```python
from build123d import *

# Parameters (mm, degrees)
SKETCH_W        = 23.25
SKETCH_H        = 34.68
PAD_DEPTH       = 10.5
SKETCH001_R     = 1.5
PAD001_DEPTH    = 2
SKETCH002_R     = 1.75
SKETCH002_R_2   = 2
SKETCH002_R_3   = 1
POCKET_DEPTH    = 1
FILLET_R        = 2.5
FILLET001_R     = 0.75
SKETCH003_W     = 5.08
SKETCH003_H     = 2.54
POCKET001_DEPTH = 5
SKETCH004_W     = 0.6
SKETCH004_H     = 0.6
SKETCH004_W_2   = 6.69
PAD002_DEPTH    = 4
SKETCH005_W     = 19.75
SKETCH005_H     = 31.18
POCKET002_DEPTH = 0.5
SKETCH006_W     = 4
SKETCH006_H     = 2.75
PAD003_DEPTH    = 2


with BuildPart() as part:
    # Sketch → Pad (new body)
    with BuildSketch(Plane.XY):
        Rectangle(SKETCH_W, SKETCH_H)
    extrude(amount=PAD_DEPTH)

    # Sketch001 (on Face5 of Pad) → Pad001 (join)
    with BuildSketch(Plane(origin=(0, 0, 0), x_dir=(1, 0, 0), z_dir=(0, 0, -1))):
        with BuildLine():
            Line((-11.625, 20.34), (-11.625, 17.34))
            Line((-11.625, 17.34), (-5.625, 17.34))
            Line((-5.625, 17.34), (-5.625, 20.34))
            ThreePointArc((-5.625, 20.34), (-8.625, 23.34), (-11.625, 20.34))
        make_face()
        with Locations((-8.625, 20.34)):
            Circle(SKETCH001_R, mode=Mode.SUBTRACT)
        with BuildLine():
            Line((5.625, 20.34), (5.625, 17.34))
            Line((5.625, 17.34), (11.625, 17.34))
            Line((11.625, 17.34), (11.625, 20.34))
            ThreePointArc((11.625, 20.34), (8.625, 23.34), (5.625, 20.34))
        make_face()
        with Locations((8.625, 20.34)):
            Circle(SKETCH001_R, mode=Mode.SUBTRACT)
    extrude(amount=-PAD001_DEPTH)

    # Sketch002 (on Face2 of Pad001) → Pocket (cut)
    with BuildSketch(Plane.XY.offset(10.5)):
        with Locations((0, 12.24)):
            Circle(SKETCH002_R)
        with Locations((0, 2.24)):
            Circle(SKETCH002_R_2)
        with Locations((0, 2.24)):
            Circle(SKETCH002_R_3, mode=Mode.SUBTRACT)
    extrude(amount=-POCKET_DEPTH, mode=Mode.SUBTRACT)

    # Fillet
    fillet_edges = [part.edges().sort_by_distance(p)[0] for p in [
        (11.625, -17.34, 6.25),
        (-11.625, -17.34, 6.25),
        (11.625, 17.34, 5.25),
        (-11.625, 17.34, 5.25),
    ]]
    fillet(fillet_edges, radius=FILLET_R)

    # Fillet001
    fillet001_edges = [part.edges().sort_by_distance(p)[0] for p in [
        (11.625, 0, 10.5),
        (10.892767, -16.607767, 10.5),
        (0, -17.34, 10.5),
        (-10.892767, -16.607767, 10.5),
        (-11.625, 0, 10.5),
        (-10.892767, 16.607767, 10.5),
        (0, 17.34, 10.5),
        (10.892767, 16.607767, 10.5),
        (-10.892767, 16.607767, 0),
        (-11.625, -18.84, 2),
        (-8.625, -23.34, 2),
        (-5.625, -18.84, 2),
        (5.625, -18.84, 2),
        (8.625, -23.34, 2),
        (11.625, -18.84, 2),
    ]]
    fillet(fillet001_edges, radius=FILLET001_R)

    # Sketch003 (on Face41 of Fillet001) → Pocket001 (cut)
    with BuildSketch(Plane(origin=(0, 17.34, 0), x_dir=(-1, 0, 0), z_dir=(0, 1, 0))):
        with Locations((-5.585, 5.25)):
            Rectangle(SKETCH003_W, SKETCH003_H)
        with BuildLine():
            ThreePointArc((1.61, 6.575), (0.285, 5.25), (1.61, 3.925))
            Line((1.61, 3.925), (7.3, 3.925))
            ThreePointArc((7.3, 3.925), (8.625, 5.25), (7.3, 6.575))
            Line((1.61, 6.575), (7.3, 6.575))
        make_face()
    extrude(amount=-POCKET001_DEPTH, mode=Mode.SUBTRACT)

    # Sketch004 (on Face55 of Pocket001) → Pad002 (join)
    with BuildSketch(Plane(origin=(0, 12.34, 0), x_dir=(-1, 0, 0), z_dir=(0, 1, 0))):
        with Locations((-7.49, 5.885)):
            Rectangle(SKETCH004_W, SKETCH004_H)
        with Locations((-6.22, 5.885)):
            Rectangle(SKETCH004_W, SKETCH004_H)
        with Locations((-4.95, 5.885)):
            Rectangle(SKETCH004_W, SKETCH004_H)
        with Locations((-3.68, 5.885)):
            Rectangle(SKETCH004_W, SKETCH004_H)
        with Locations((4.455, 5.25)):
            Rectangle(SKETCH004_W_2, SKETCH004_H)
    extrude(amount=PAD002_DEPTH)

    # Sketch005 (on Face9 of Pad002) → Pocket002 (cut)
    with BuildSketch(Plane(origin=(0, 0, 0), x_dir=(1, 0, 0), z_dir=(0, 0, -1))):
        Rectangle(SKETCH005_W, SKETCH005_H)
    extrude(amount=-POCKET002_DEPTH, mode=Mode.SUBTRACT)

    # Sketch006 (on Face24 of Pocket002) → Pad003 (join)
    with BuildSketch(Plane.YZ.offset(11.625)):
        with Locations((-10.34, 5.375)):
            Rectangle(SKETCH006_W, SKETCH006_H)
    pad003 = extrude(amount=PAD003_DEPTH)

    # Mirrored: Pad003 across YZ
    add(pad003.mirror(Plane.YZ))


solid = part.part
```
Here's how the part is built. I have some questions about the finished solid (model axes, mm). A direction names the side the tool comes from. Round coordinates to 2 decimals unless told otherwise and drop trailing zeros. Write each loop counter-clockwise with the first axis right and the second up, starting at its lowest first coordinate (ties: lowest second). Pieces come first, ordered by that corner, then holes.
Q1. If we section it at A-A on z = 7.25: Write out the boundary of the cut face in (x, y) (3 decimals).
Q2. If we section it at B-B on y = 2.24: Write out the boundary of the cut face in (x, z) (3 decimals), plus the area to 3 significant figures.
Q3. Which directions (+Z, -Z, +X, -X, +Y, -Y) give clear straight access to the entire face, cutting with the end or side of a thin tool? Please do faces 5 (the flat face through (-13, -12.34, 5)), 6 (the cylindrical face through (-0.38, 10.53, 10.01)), 7 (the flat face through (13, -8.34, 5)), 8 (the flat face through (8.125, 15, 5)).
Q4. Please list where these lines run through material, in increasing order: probe 1 along X at (y, z) = (-20.34, 0.8) (3 decimals); probe 2 along Y at (x, z) = (0, 9.8); probe 3 along Z at (x, y) = (4.5, 13).
Q5. Will these pins go through, and if not, where does the flat tip stop? P1, Ø0.6, axis at y = -19.5, z = 1, coming from the +X side (3 decimals); P2, Ø0.6, axis at y = -19.5, z = 1, coming from the -X side (3 decimals); P3, Ø0.5, axis at x = 7.5, y = 15, coming from the -Z side.
Q6. If we mould it in two halves opening along X, with no side actions, what happens to faces 1 (the flat face through (13.625, -10, 5)), 2 (the flat face through (-4, 15, 3.925)), 3 (the flat face through (-13, -10, 6.75)), 4 (the cylindrical face through (8.69, -23.34, 1))? For each: +X half, -X half, draft (parallel to the pull), parting line (faces both ways), or undercut.
Answer below:
1. outline: (-11.625, -14.84) arc R2.5 ccw to (-9.125, -17.34) - (9.125, -17.34) arc R2.5 ccw to (11.625, -14.84) - (11.625, 14.84) arc R2.5 ccw to (9.125, 17.34) - (-9.125, 17.34) arc R2.5 ccw to (-11.625, 14.84) - close
2. outline: (-11.625, 0.75) arc R0.75 ccw to (-10.875, 0) - (-9.875, 0) - (-9.875, 0.5) - (9.875, 0.5) - (9.875, 0) - (10.875, 0) arc R0.75 ccw to (11.625, 0.75) - (11.625, 9.75) arc R0.75 ccw to (10.875, 10.5) - (2, 10.5) - (2, 9.5) - (1, 9.5) - (1, 10.5) - (-1, 10.5) - (-1, 9.5) - (-2, 9.5) - (-2, 10.5) - (-10.875, 10.5) arc R0.75 ccw to (-11.625, 9.75) - close
2. area: 232 mm2
3. face 5: +Z, -Z, -X, -Y
3. face 6: +Z
3. face 7: +Z, -Z, +X, +Y
3. face 8: +Y
4. probe 1: x = -11.625 to -10.125, -7.125 to -5.625, 5.625 to 7.125, 10.125 to 11.625
4. probe 2: y = -17.34 to 0.24, 1.24 to 3.24, 4.24 to 10.49, 13.99 to 17.34
4. probe 3: z = 0.5 to 3.98, 6.52 to 10.5
5. P1: stops at x = 11.625
5. P2: stops at x = -11.625
5. P3: stops at z = 0.5
6. face 1: +X half
6. face 2: undercut
6. face 3: draft
6. face 4: undercut
